Check sheet for the drawn part. Datum: minimum x, y, z corner. Units: mm. A direction names the side the tool comes from. Coordinates: 2 decimals unless noted, no trailing zeros. Write each loop counter-clockwise with the first axis right and the second up, starting at its lowest first coordinate (ties: lowest second). Pieces come first, ordered by that corner, then holes. Notation, with made-up numbers: (23.5, 55.5) - (36.5, 55.5) arc R17 ccw to (36.5, 74.5) - close; hole circle Ø2 at (-9, -5.75). An arc over 180 degrees is marked (long way). Use one line per item in the form item = value. Start each with the question number.
1. Scan lines: line 1 along X through (y, z) = (1.5, 10.75); line 2 along Z through (x, y) = (22, 23); line 3 along Z through (x, y) = (11.5, 2). Record each from-to range of solid material in increasing order.
2. Cross-section at B-B on y = 18.5. Record the boundary of the cut face in (x, z), then the cut area to 3 significant figures.
3. Cross-section at C-C on x = 26. Record the boundary of the cut face in (y, z).
4. Tool access check on the marked faces 1, 2, 3, 4 and 5. Record the directions out of +Z, -Z, +X, -X, +Y, -Y that give a thin tool (end or side, any length) a straight path to the whole face; none if there is none.
5. Go/stop test with flat-tipped pins: pin 1 Ø5 at (x, z) = (4.5, 3) entering from -Y; pin 2 Ø4 at (x, y) = (3, 17) entering from +Z; pin 3 Ø10 at (y, z) = (20.5, 6) entering from -X. Record where each tip stops, or that it passes through.
6. Cross-section at A-A on z = 3. Record the boundary of the cut face in (x, y), then the cut area to 4 significant figures.
7. Cross-section at D-D on x = 8.5. Record the boundary of the cut face in (y, z).
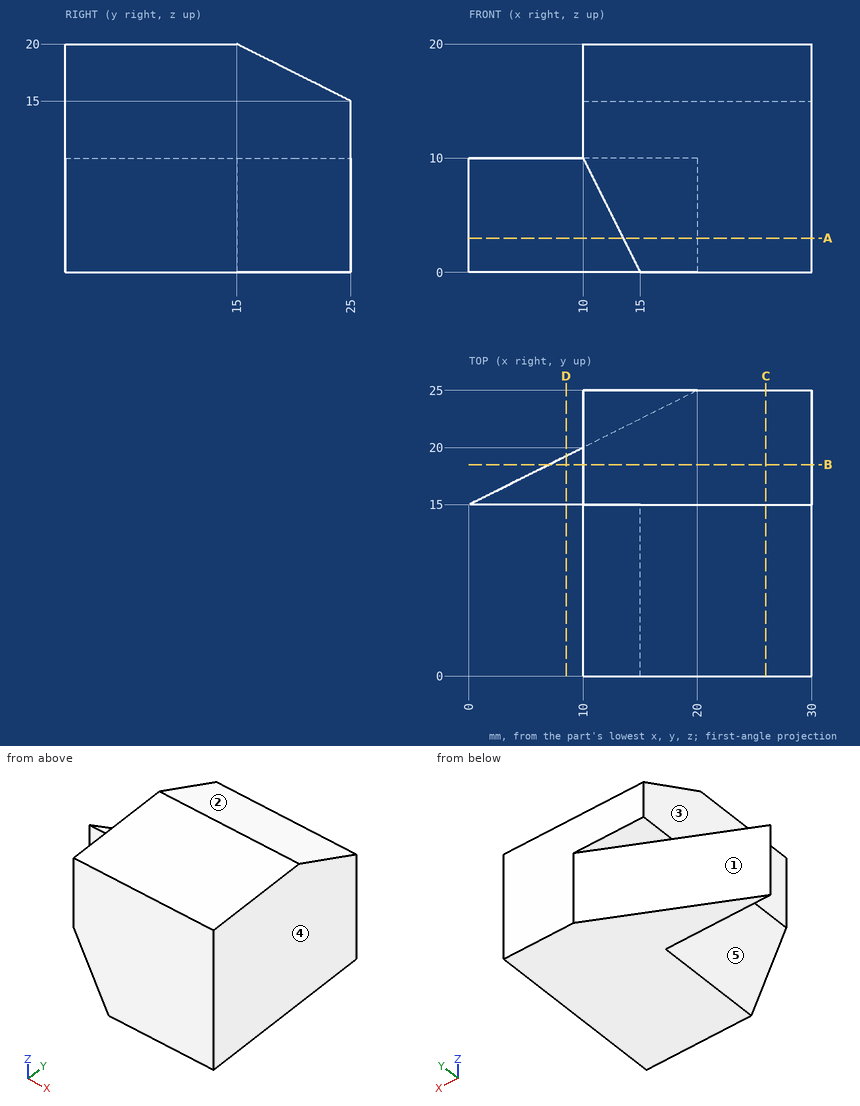
Final values:
q1.line_1 = 10 to 30
q1.line_2 = 0 to 16
q1.line_3 = 7 to 20
q2.outline = (7, 0) - (30, 0) - (30, 18.25) - (10, 18.25) - (10, 10) - (7, 10) - close
q2.area = 395 mm²
q3.outline = (0, 0) - (25, 0) - (25, 15) - (15, 20) - (0, 20) - close
q4.face_1 = -Z, -X, +Y
q4.face_2 = +Z, +X, -X, +Y
q4.face_3 = +Z, -X, +Y, -Y
q4.face_4 = +Z, -Z, +X, +Y, -Y
q4.face_5 = -Z, -X, -Y
q5.pin_1 = 15
q5.pin_2 = 10
q5.pin_3 = 1
q6.outline = (0, 15) - (13.5, 15) - (13.5, 0) - (30, 0) - (30, 25) - (20, 25) - close
q6.area = 447.5 mm²
q7.outline = (15, 0) - (19.25, 0) - (19.25, 10) - (15, 10) - close
